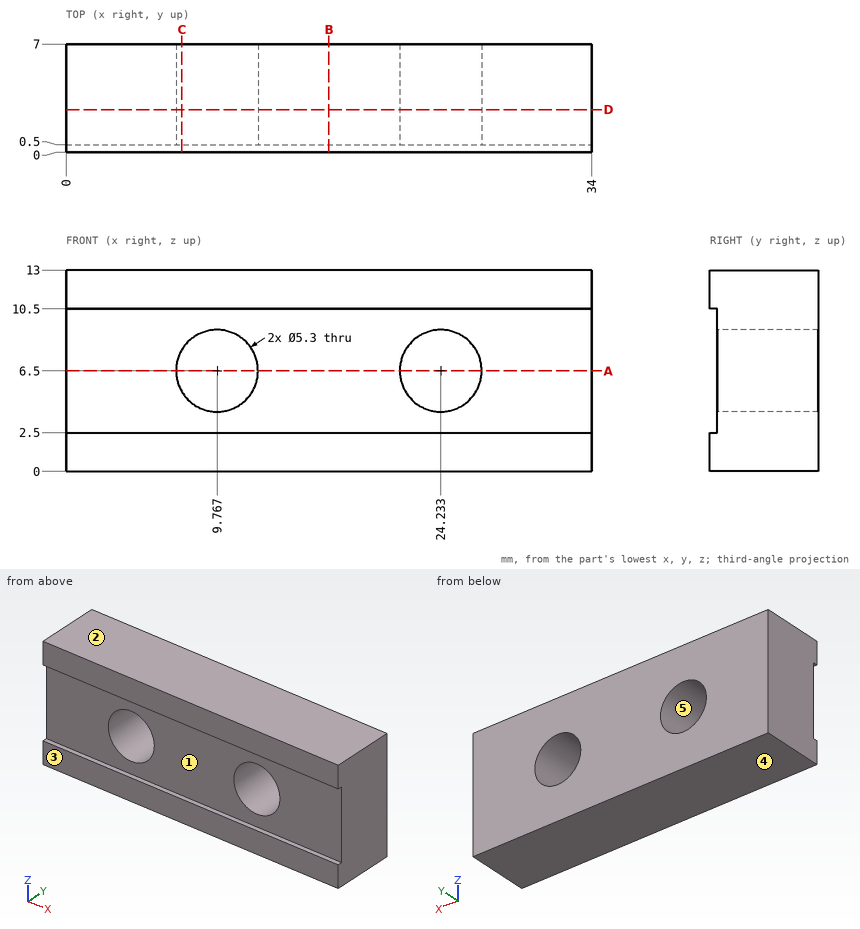
Geometry: see drawing. Coordinates: mm, zero at the bounding-box minimum. A direction names the side the tool comes from. Coordinates: 2 decimals unless noted, no trailing zeros. Write each loop counter-clockwise with the first axis right and the second up, starting at its lowest first coordinate (ties: lowest second). Pieces come first, ordered by that corner, then holes. Notation, with made-up numbers: (3, 54.25) - (44, 54.25) arc R25 ccw to (44, 67.25) - close; hole circle Ø10 at (9, 0). An arc over 180 degrees is marked (long way). Put each result on its own line as item: value. Start each with the question number.
1) Cut plane D-D (y = 2.75). Return the cut outline in (x, z), plus the area to 3 significant figures.
2) Contact query for flat-ended pins moving along their axis: pin 1 (3 mm diameter, centred on y = 4, z = 11, fed in from -X); pin 2 (6 mm diameter, centred on x = 9.77, z = 6.5, fed in from -Y); pin 3 (4 mm diameter, centred on x = 24.23, z = 6.5, fed in from +Y). Output: stop coordinate, or through.
3) Cut plane C-C (x = 7.5). Return the cut outline in (y, z).
4) Cut plane B-B (x = 17). Return the cut outline in (y, z), plus the area to 3 significant figures.
5) Cut plane A-A (z = 6.5). Return the cut outline in (x, y).
6) Reachability of the marked faces 1 and 2 from +Z, -Z, +X, -X, +Y, -Y: full face, straight path, thin tool, end or side. Return the list, or none.
7) Ray query, L1, parallel to X at y = 2, z = 6.5; L2, parallel to X at y = 1, z = 6 (1 decimal); L3, parallel to Z at x = 8, y = 1.25 (1 decimal). Return the intervals inside material, ascending.
8) Mould query, pull axis Z, two halves, no side actions, for the marked faces 3, 4 and 5. Classes: pulls with the +Z half, pulls with the -Z half, needs draft (parallel to the pull), parting line crosses it, or undercut.
Resolved:
1. outline: (0, 0) - (34, 0) - (34, 13) - (0, 13) - close; hole circle Ø5.3 at (9.77, 6.5); hole circle Ø5.3 at (24.23, 6.5)
1. area: 398 mm2
2. pin 1: stops at x = 0
2. pin 2: stops at y = 0.5
2. pin 3: passes through
3. outline: (0, 0) - (7, 0) - (7, 5.13) - (0.5, 5.13) - (0.5, 2.5) - (0, 2.5) - close; (0, 10.5) - (0.5, 10.5) - (0.5, 7.87) - (7, 7.87) - (7, 13) - (0, 13) - close
4. outline: (0, 0) - (7, 0) - (7, 13) - (0, 13) - (0, 10.5) - (0.5, 10.5) - (0.5, 2.5) - (0, 2.5) - close
4. area: 87.0 mm2
5. outline: (0, 0.5) - (7.12, 0.5) - (7.12, 7) - (0, 7) - close; (12.42, 0.5) - (21.58, 0.5) - (21.58, 7) - (12.42, 7) - close; (26.88, 0.5) - (34, 0.5) - (34, 7) - (26.88, 7) - close
6. face 1: +X, -X, -Y
6. face 2: +Z, +X, -X, +Y, -Y
7. L1: x = 0 to 7.12, 12.42 to 21.58, 26.88 to 34
7. L2: x = 0 to 7.2, 12.4 to 21.6, 26.8 to 34
7. L3: z = 0 to 4.5, 8.5 to 13
8. face 3: needs draft
8. face 4: pulls with the -Z half
8. face 5: undercut
